from build123d import *

# Parameters (mm, degrees)
F1_DEPTH = 19.05
F2_SIZE  = 19.04999
F3_SIZE  = 19.04999


# Not quite as in the source:
# - a fillet or chamfer is up to 0.001 mm smaller than in the source, because OpenCascade refuses the exact size


with BuildPart() as f1:
    # F0 (on Top) → F1 (new body)
    with BuildSketch(Plane.XY):
        Polygon((-120.9837489087, -207.2259), (120.9837489087, -67.5259), (120.9837489087, 207.2259), (-120.9837489087, 67.5259), align=None)
    extrude(amount=F1_DEPTH)

    # F2 (size 19.05 in the source; OpenCascade refuses exactly that, so slightly less here)
    f2_edges = [f1.edges().sort_by_distance(p)[0] for p in [
        (-120.983749, -69.85, 19.05),
    ]]
    chamfer(f2_edges, length=F2_SIZE)

    # F3 (size 19.05 in the source; OpenCascade refuses exactly that, so slightly less here)
    f3_edges = [f1.edges().sort_by_distance(p)[0] for p in [
        (120.983749, 69.85, 19.05),
    ]]
    chamfer(f3_edges, length=F3_SIZE)


solid = f1.part
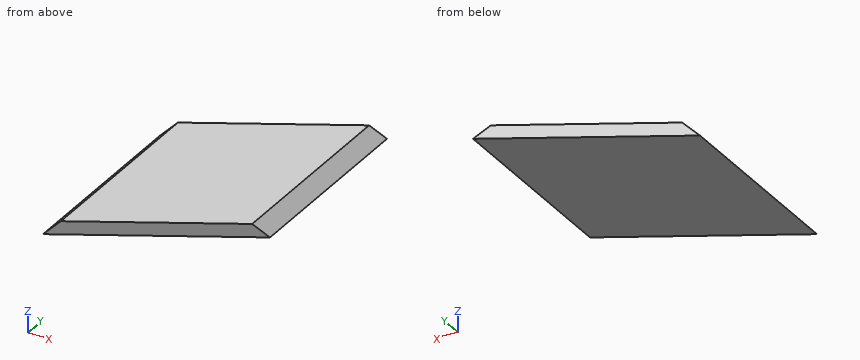
Verification items for the finished model (mm, model axes). Round coordinates to 2 decimals unless told otherwise and drop trailing zeros. Order: outer loops, then holes, each group sorted by start corner. A loop starts at its lowest first (then second) coordinate and runs counter-clockwise, first axis right, second up. Notation, with made-up numbers: (76.5, 71.5) -> (128.5, 71.5) arc R18 ccw to (128.5, 99.5) -> close; hole circle Ø11 at (82, 11.5). An arc over 180 degrees is marked (long way). Put each result on its own line as item: value.
1) Material ranges on line 1 (Y direction, x = 48, z = 1); line 2 (X direction, y = -159, z = 16.75); line 3 (X direction, y = -154, z = 12.25), recorded low to high.
Final values:
line 1: y = -109.66 to 165.09
line 2: x = -104.23 to -37.45
line 3: x = -108.73 to -28.79
2) Depth check by flat-ended pin: pin 1 (1 mm diameter, centred on y = 5.5, z = 13.5, fed in from +X); pin 2 (2 mm diameter, centred on x = -79, y = 20, fed in from -Z); pin 3 (8 mm diameter, centred on x = -65, z = 11, fed in from -Y); pin 4 (3 mm diameter, centred on y = -57.5, z = 16, fed in from +X). Enter the tip coordinate at first touch or a pass-through.
Final values:
pin 1: stops at x = 107.98
pin 2: stops at z = 0
pin 3: stops at y = -177.21
pin 4: stops at x = 106.48
3) Section check C-C (x = 49.5). Record the cut outline in (y, z).
Final values:
outline: (-108.8, 0) -> (165.95, 0) -> (165.95, 19.05) -> (-108.8, 19.05) -> close
4) Section check B-B (z = 13.75). Record the cut outline in (x, y), then the cut area to 3 significant figures.
Final values:
outline: (-107.23, -199.29) -> (107.23, -75.46) -> (107.23, 199.29) -> (-107.23, 75.46) -> close
area: 58,900 mm^2
